The model under review builds one solid part; all positions refer to its coordinate system, in mm. Face numbers are marked on the shaded views. A direction names the side the tool comes from. Coordinates: 2 decimals unless noted, no trailing zeros. Loops run counter-clockwise (first coordinate to the right, second up) from the corner with the lowest first, then second, coordinate; pieces in that order, holes last. Notation, with made-up numbers: M 56,-34.75 L 76,-34.75 A34 cw 76,3.25 Z; hole C -11,20 d2. An arc over 180 degrees is marked long. Use CSV: the item, a comma, the result in double quotes. Start each with the question number.
from build123d import *

# Parameters (mm, degrees)
SKETCH1_W           = 10
SKETCH1_H           = 10
BOSS_EXTRUDE1_DEPTH = 4
SKETCH2_R           = 4
BOSS_EXTRUDE2_DEPTH = 3
CUT_EXTRUDE1_DEPTH  = 1.5


with BuildPart() as part:
    # Sketch1 → Boss-Extrude1 (new body)
    with BuildSketch(Plane.XY):
        with Locations((5, -5)):
            Rectangle(SKETCH1_W, SKETCH1_H)
    extrude(amount=BOSS_EXTRUDE1_DEPTH)

    # Sketch2 → Boss-Extrude2 (add)
    with BuildSketch(Plane.XY.offset(4)):
        with Locations((5, -5)):
            Circle(SKETCH2_R)
    extrude(amount=BOSS_EXTRUDE2_DEPTH)

    # Sketch3 → Cut-Extrude1 (cut)
    with BuildSketch(Plane.XY.offset(7)):
        Polygon((4, -4), (4, -2.25), (6, -2.25), (6, -4), (7.75, -4), (7.75, -6), (6, -6), (6, -7.75), (4, -7.75), (4, -6), (2.25, -6), (2.25, -4), align=None)
    extrude(amount=-CUT_EXTRUDE1_DEPTH, mode=Mode.SUBTRACT)


solid = part.part
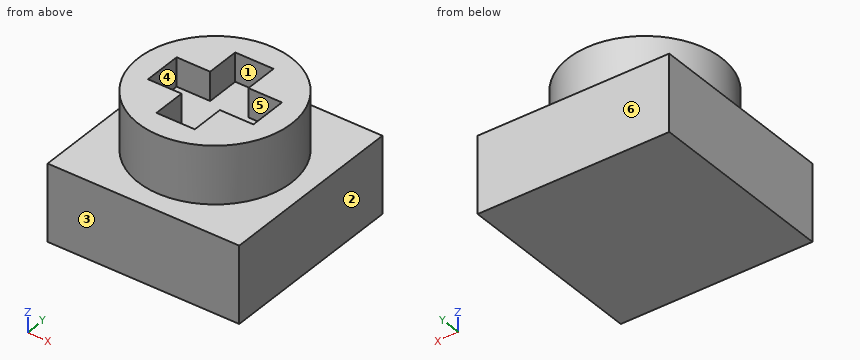
1. Add section A-A (z = 6). Write out the cut boundary in (x, y), plus the area to 3 significant figures.
2. Draft analysis for pull direction Y (two halves, no side actions). For the marked faces 1, 2, 3 and 4, state which applies: released by +Y, released by -Y, zero draft, split by the parting line, or undercut.
3. Insertion check: pin 1 Ø1.6 at (x, z) = (7, 6.5) entering from +Y; pin 2 Ø1.6 at (y, z) = (-6.5, 6.5) entering from +X; pin 3 Ø1.6 at (x, z) = (7, 6) entering from -Y. Each pin has a flat end and moves straight along its axis. Give the tip position at first contact, or say it passes through.
4. Add section C-C (x = 5). Write out the cut boundary in (y, z), plus the area to 4 significant figures.
5. Add section D-D (y = -8.75). Write out the cut boundary in (x, z).
6. Add section B-B (y = -5). Write out the cut boundary in (x, z), plus the area to 4 significant figures.
7. For the marked faces 5 and 6, list the 3-axis set-ups (+Z, -Z, +X, -X, +Y, -Y) from which the entire face can be reached by the end or side of a thin tool; tool diameter is ignored.
8. To check wall thickness, follow line 1 along Z through (x, y) = (5, -4); line 2 along Z through (x, y) = (5.5, -9.5); line 3 along Y through (x, z) = (3, 6.75). State the ranges of each line that lie inside material, in increasing order.
Solved:
1,outline,"C 5,-5 d8; hole M 2.25,-6 L 4,-6 L 4,-7.75 L 6,-7.75 L 6,-6 L 7.75,-6 L 7.75,-4 L 6,-4 L 6,-2.25 L 4,-2.25 L 4,-4 L 2.25,-4 Z"
1,area,"32.3 mm^2"
2,face 1,"undercut"
2,face 2,"zero draft"
2,face 3,"released by -Y"
2,face 4,"undercut"
3,pin 1,"stops at y = -1.18"
3,pin 2,"stops at x = 8.94"
3,pin 3,"stops at y = -8.82"
4,outline,"M -10,0 L 0,0 L 0,4 L -1,4 L -1,7 L -2.25,7 L -2.25,5.5 L -7.75,5.5 L -7.75,7 L -9,7 L -9,4 L -10,4 Z"
4,area,"55.75 mm^2"
5,outline,"M 0,0 L 10,0 L 10,4 L 6.39,4 L 6.39,7 L 3.61,7 L 3.61,4 L 0,4 Z"
6,outline,"M 0,0 L 10,0 L 10,4 L 9,4 L 9,7 L 7.75,7 L 7.75,5.5 L 2.25,5.5 L 2.25,7 L 1,7 L 1,4 L 0,4 Z"
6,area,"55.75 mm^2"
7,face 5,"+Z"
7,face 6,"+Z, -Z, +X, -X, +Y"
8,line 1,"z = 0 to 5.5"
8,line 2,"z = 0 to 4"
8,line 3,"y = -8.46 to -6, -4 to -1.54"
